Source: CAD feature listing. Evaluate the final solid. Frame: model axes, mm. A direction names the side the tool comes from. Round coordinates to 2 decimals unless told otherwise and drop trailing zeros. Loops run counter-clockwise (first coordinate to the right, second up) from the corner with the lowest first, then second, coordinate; pieces in that order, holes last.
Item 1: Section query B-B on x = 26. Return loops of the section in (y, z), then the cut area to 3 significant figures.
Item 2: First-contact query: P1, Ø8, axis at y = 1.5, z = -17.5, coming from the +X side; P2, Ø8, axis at x = -25, z = 0, coming from the -Y side; P3, Ø10, axis at x = -25.5, y = 4.5, coming from the -Z side; P4, Ø8, axis at y = 4, z = -9.5, coming from the +X side. Flat tips, straight axial feed; report the tip coordinate or a pass-through.
Item 3: Section query A-A on z = 0. Return loops of the section in (x, y), then the cut area to 3 significant figures.
Item 4: Ray query, L1, parallel to X at y = 3, z = 0; L2, parallel to Z at x = -25, y = 1.5; L3, parallel to X at y = 5, z = -18.5. Return the intervals inside material, ascending.
Item 5: Section query D-D on y = 7.25. Return loops of the section in (x, z).
Item 6: Section query C-C on z = -18. Return loops of the section in (x, y).
Item 7: Access query for faces 4 (the flat face through (9, 0, -20)), 5 (the cylindrical face through (7, 9, -20)), 6 (the cylindrical face through (-7, -9, -20)). Directions: +Z, -Z, +X, -X, +Y, -Y. A direction counts if a zero-diameter tool reaches every point of the face in a straight line with its end or side. Return the directions, or none.
Item 8: Pull-direction query (Z, two-part tool) for faces 1 (the cylindrical face through (-31.445, 0.14, 0.846)), 2 (the cylindrical face through (-8, 8, -20)), 3 (the flat face through (-17, 0, -10)); classes: released by +Z, released by -Z, zero draft, split by the parting line, or undercut.
Autodesk Inventor part; units mm, degrees
sketch "Skizze1" plane through (0, 0, 0) normal (0, 1, 0) x (-1, 0, 0)
  line L0 (25, 10) -> (-25, 10)
  line L1 (-35, 0) -> (-35, 0)
  line L2 (-25, -10) -> (25, -10)
  line L3 (35, 0) -> (35, 0)
  line L4 (51.8995, 0) -> (-51.8995, 0)
  line L5 (0, -16.8995) -> (0, 16.8995)
  arc A0 (35, 8) -> (33, 10) centre (33, 8) ccw
  arc A1 (33, -10) -> (35, -8) centre (33, -8) ccw
  arc A2 (-33, 10) -> (-35, 8) centre (-33, 8) ccw
  arc A3 (-35, -8) -> (-33, -10) centre (-33, -8) ccw
  arc A4 (35, 0) -> (25, 10) centre (25, 0) ccw
  arc A5 (25, -10) -> (35, 0) centre (25, 0) ccw
  arc A6 (-25, 10) -> (-35, 0) centre (-25, 0) ccw
  arc A7 (-35, 0) -> (-25, -10) centre (-25, 0) ccw
  point P0 (0, 0)
  point P1 (-35, -10)
  point P2 (-35, 10)
  point P3 (35, -10)
  point P4 (-35, 0)
  dimension "d0" = 70
  dimension "d1" = 20
  dimension "d2" = 2
  dimension "d3" = 10
extrude "Extrusion1" add sketch "Skizze1" along normal mid plane 20
ref_plane "Arbeitsebene1" through (0, -10, 0) normal (0, 1, 0) x (-1, 0, 0)
sketch "Skizze3" plane through (0, -10, 0) normal (0, -1, 0) x (1, 0, 0)
  arc A0 (-25, 10) -> (-25, -10) centre (-25, 0) ccw
  arc A1 (25, -10) -> (25, 10) centre (25, 0) ccw
  point P0 (0, 0)
hole "Bohrung1" at (-25, -10, 0) at (25, -10, 0) direction (0, 1, 0) diameter 6.756 end through all counterbore diameter 13 counterbore depth 20
ref_plane "Arbeitsebene2" through (0, 0, -10) normal (0, 0, 1) x (1, 0, 0)
sketch "Skizze4" plane through (0, 0, -10) normal (0, 0, 1) x (1, 0, 0)
  line L0 (9, 10) -> (-9, 10)
  line L1 (-9, 10) -> (-9, -10)
  line L2 (-9, -10) -> (9, -10)
  line L3 (9, -10) -> (9, 10)
  line L4 (0, -26) -> (0, 16)
  line L5 (-49, 0) -> (49, 0)
  dimension "d15" = 18
  dimension "d16" = 20
extrude "Extrusion2" add sketch "Skizze4" against normal blind 20
fillet "Rundung1" radius 5 4 edges at (-9, -10, -20) (9, -10, -20) (9, 10, -20) (-9, 10, -20)
properties part number "Schlitten1"
Data:
1. outline: (-10, -9.95) - (10, -9.95) - (10, -6.42) - (-10, -6.42) - close; (-10, 6.42) - (10, 6.42) - (10, 9.95) - (-10, 9.95) - close
1. area: 141 mm2
2. P1: stops at x = 9
2. P2: passes through
2. P3: stops at z = -10
2. P4: stops at x = 33.35
3. outline: (-35, -10) - (-31.5, -10) - (-31.5, 10) - (-35, 10) - close; (-18.5, -10) - (18.5, -10) - (18.5, 10) - (-18.5, 10) - close; (31.5, -10) - (35, -10) - (35, 10) - (31.5, 10) - close
3. area: 880 mm2
4. L1: x = -35 to -31.5, -18.5 to 18.5, 31.5 to 35
4. L2: z = -10 to -6.5, 6.5 to 10
4. L3: x = -9 to 9
5. outline: (-25, -10) - (-8.47, -10) - (-8.47, -30) - (8.47, -30) - (8.47, -10) - (25, -10) arc R10 ccw to (25, 10) - (-25, 10) arc R10 ccw to start; hole circle Ø13 at (-25, 0); hole circle Ø13 at (25, 0)
6. outline: (-9, -5) arc R5 ccw to (-4, -10) - (4, -10) arc R5 ccw to (9, -5) - (9, 5) arc R5 ccw to (4, 10) - (-4, 10) arc R5 ccw to (-9, 5) - close
7. face 4: -Z, +X, +Y, -Y
7. face 5: -Z, +X, +Y
7. face 6: -Z, -X, -Y
8. face 1: undercut
8. face 2: zero draft
8. face 3: released by -Z
